CAD build for the part. Positions are in the model's coordinates, mm. Round coordinates to 2 decimals unless told otherwise and drop trailing zeros. Order: outer loops, then holes, each group sorted by start corner. A loop starts at its lowest first (then second) coordinate and runs counter-clockwise, first axis right, second up.
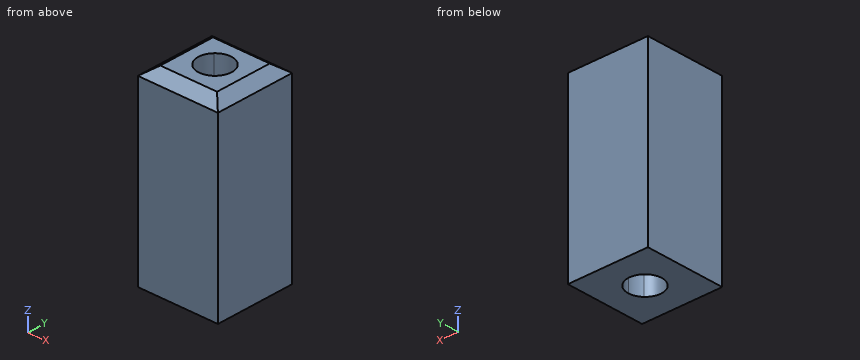
```python
from build123d import *

# Parameters (mm, degrees)
F0_W     = 304.8
F0_H     = 304.8
F1_DEPTH = 711.2
F2_SIZE2 = 44.45
F2_SIZE  = 31.75
F4_DEPTH = 711.201


with BuildPart() as f1:
    # F0 (on Top) → F1 (new body)
    with BuildSketch(Plane.XY):
        with Locations((-152.4, 152.4)):
            Rectangle(F0_W, F0_H)
    extrude(amount=F1_DEPTH)

    # F2
    f2_edges = [f1.edges().sort_by_distance(p)[0] for p in [
        (-152.4, 0, 711.2),
        (0, 152.4, 711.2),
        (-152.4, 304.8, 711.2),
        (-304.8, 152.4, 711.2),
    ]]
    chamfer(f2_edges, length=F2_SIZE, length2=F2_SIZE2)

    # F3 (on face) → F4 (cut, through all)
    with BuildSketch(Plane.XY.offset(711.2)):
        with BuildLine():
            ThreePointArc((-88.9, 152.4), (-128.099602, 211.06635), (-197.301281, 197.301281))
            Line((-197.301281, 197.301281), (-107.498719, 107.498719))
            ThreePointArc((-107.498719, 107.498719), (-93.73365, 128.099602), (-88.9, 152.4))
        make_face()
        with BuildLine():
            Line((-107.498719, 107.498719), (-197.301281, 197.301281))
            ThreePointArc((-197.301281, 197.301281), (-197.301281, 107.498719), (-107.498719, 107.498719))
        make_face()
    extrude(amount=-F4_DEPTH, mode=Mode.SUBTRACT)


solid = f1.part
```
1. Cut at A-A, the plane x = -152.4. Write the cut outline in (y, z).
2. Pin check, flat tip, straight feed: P1, Ø2, axis at x = -231.5, y = 89.5, coming from the -Z side. Stop position of the tip, or through.
3. Drill centre lines: line 1 (Y direction, x = -150, z = 124.5); line 2 (Y direction, x = -103, z = 267); line 3 (X direction, y = 141, z = 640.5). Where is each one in solid material? Low to high.
4. Cut at B-B, the plane z = 444. Write the cut outline in (x, y), and give its area (3 significant figures).
Outcome:
1. outline: (0, 0) - (88.9, 0) - (88.9, 711.2) - (44.45, 711.2) - (0, 679.45) - close; (215.9, 0) - (304.8, 0) - (304.8, 679.45) - (260.35, 711.2) - (215.9, 711.2) - close
2. P1: stops at z = 0
3. line 1: y = 0 to 88.95, 215.85 to 304.8
3. line 2: y = 0 to 112.5, 192.3 to 304.8
3. line 3: x = -304.8 to -214.87, -89.93 to 0
4. outline: (-304.8, 0) - (0, 0) - (0, 304.8) - (-304.8, 304.8) - close; hole (-107.5, 107.5) arc R63.5 ccw to (-88.9, 152.4) arc R63.5 ccw (long way) to start
4. area: 80,200 mm2
